from build123d import *

# Parameters (mm, degrees)
SKETCH1_W           = 120
SKETCH1_H           = 70
SKETCH1_R           = 2.5
SKETCH1_R_2         = 1.9
SKETCH1_W_2         = 5
SKETCH1_H_2         = 30
BOSS_EXTRUDE1_DEPTH = 10
CHAMFER1_SIZE       = 10
SKETCH3_W           = 10
SKETCH3_H           = 20
BOSS_EXTRUDE2_DEPTH = 3
FILLET1_R           = 1.5


with BuildPart() as part:
    # Sketch1 → Boss-Extrude1 (new body)
    with BuildSketch(Plane(origin=(0, 0, 0), x_dir=(1, 0, 0), z_dir=(0, 1, 0))):
        Rectangle(SKETCH1_W, SKETCH1_H)
        with Locations(Location((-50, 25, 0), (0, 0, 270))):
            Circle(SKETCH1_R, mode=Mode.SUBTRACT)
        with Locations(Location((-50, -25, 0), (0, 0, 90))):
            Circle(SKETCH1_R, mode=Mode.SUBTRACT)
        with Locations(Location((8, 0, 0), (0, 0, 270))):
            Circle(SKETCH1_R_2, mode=Mode.SUBTRACT)
        Polygon((18, 23.5), (18, 4.5), (3, 4.5), (3, -4.5), (18, -4.5), (18, -23.5), (-20, -23.5), (-20, 23.5), align=None, mode=Mode.SUBTRACT)
        with Locations((45, 0)):
            Rectangle(SKETCH1_W_2, SKETCH1_H_2, mode=Mode.SUBTRACT)
    extrude(amount=BOSS_EXTRUDE1_DEPTH)

    # Chamfer1
    chamfer1_edges = [part.edges().sort_by_distance(p)[0] for p in [
        (45, 10, 15),
        (45, 10, -15),
    ]]
    chamfer(chamfer1_edges, length=CHAMFER1_SIZE - 0.0001)  # a hair under: the kernel refuses the full size

    # Sketch3 → Boss-Extrude2 (add)
    with BuildSketch(Plane(origin=(0, 10, 0), x_dir=(1, 0, 0), z_dir=(0, 1, 0))):
        with Locations((30, -35)):
            Rectangle(SKETCH3_W, SKETCH3_H)
    extrude(amount=BOSS_EXTRUDE2_DEPTH)

    # Fillet1
    fillet1_edges = [part.edges().sort_by_distance(p)[0] for p in [
        (25, 13, 35),
        (35, 13, 35),
        (30, 13, 25),
        (35, 10, 30),
        (30, 10, 25),
        (25, 10, 30),
    ]]
    fillet(fillet1_edges, radius=FILLET1_R - 0.0001)  # a hair under: the kernel refuses the full size


solid = part.part
Input: part model. Units: mm. Frame: model coordinates. A direction names the side the tool comes from. Coordinates: 2 decimals unless noted, no trailing zeros. Loops run counter-clockwise (first coordinate to the right, second up) from the corner with the lowest first, then second, coordinate; pieces in that order, holes last.
(1) Section C-C on x = 12.5. Return the cut outline in (y, z).
(2) Section A-A on x = -1. Return the cut outline in (y, z), then the cut area to 3 significant figures.
(3) Pull-direction query (X, two-part tool) for faces 4 (the face through (-60, 5, 0)), 5 (the face through (30, 10, 40)), 6 (the face through (18, 5, -14)); classes: released by +X, released by -X, zero draft, split by the parting line, or undercut.
(4) Material intervals for probe 1 along X at (y, z) = (7.75, 0); probe 2 along X at (y, z) = (4.25, -16.5); probe 3 along Z at (x, y) = (-7, 3.25), sorted ascending.
(5) First-contact query: pin 1 Ø3 at (x, z) = (8, 0) entering from +Y; pin 2 Ø8 at (x, z) = (30.5, 41.5) entering from -Y; pin 3 Ø0.5 at (y, z) = (10.5, 35.5) entering from -X; pin 4 Ø10 at (x, z) = (13, -2) entering from +Y. Flat tips, straight axial feed; report the tip coordinate or a pass-through.
(6) Set-up query: faces 1 (the face through (10, 5, 4.5)), 2 (the face through (45, 5, -20)), 3 (the face through (60, 5, 0)). Return all of +Z, -Z, +X, -X, +Y, -Y with unobstructed straight access to the full face (end or side cutting, diameter ignored); none if empty.
(7) Section B-B on z = 6.5. Return the cut outline in (x, y), then the cut area to 3 significant figures.
(8) Section D-D on y = 1.5. Return the cut outline in (x, z).
Data:
1. outline: (0, -35) - (10, -35) - (10, -23.5) - (0, -23.5) - close; (0, -4.5) - (10, -4.5) - (10, 4.5) - (0, 4.5) - close; (0, 23.5) - (10, 23.5) - (10, 35) - (0, 35) - close
2. outline: (0, -35) - (10, -35) - (10, -23.5) - (0, -23.5) - close; (0, 23.5) - (10, 23.5) - (10, 35) - (0, 35) - close
2. area: 230 mm2
3. face 4: released by -X
3. face 5: zero draft
3. face 6: undercut
4. probe 1: x = -60 to -20, 3 to 6.1, 9.9 to 42.5, 47.5 to 60
4. probe 2: x = -60 to -20, 18 to 42.5, 47.5 to 60
4. probe 3: z = -35 to -23.5, 23.5 to 35
5. pin 1: passes through
5. pin 2: stops at y = 10
5. pin 3: stops at x = 25
5. pin 4: stops at y = 10
6. face 1: +Y, -Y
6. face 2: +Y
6. face 3: +Z, -Z, +X, +Y, -Y
7. outline: (-60, 0) - (-20, 0) - (-20, 10) - (-60, 10) - close; (18, 0) - (42.5, 0) - (42.5, 10) - (18, 10) - close; (47.5, 0) - (60, 0) - (60, 10) - (47.5, 10) - close
7. area: 770 mm2
8. outline: (-60, -35) - (60, -35) - (60, 35) - (-60, 35) - close; hole circle Ø5 at (-50, -25); hole circle Ø5 at (-50, 25); hole (-20, -23.5) - (18, -23.5) - (18, -4.5) - (3, -4.5) - (3, 4.5) - (18, 4.5) - (18, 23.5) - (-20, 23.5) - close; hole circle Ø3.8 at (8, 0); hole (42.5, -16.5) - (47.5, -16.5) - (47.5, 16.5) - (42.5, 16.5) - close
